from build123d import *

# Parameters (mm, degrees)
SKETCH_1_R          = 25
EXTRUDE_1_DEPTH     = 80
CUT_EXTRUDE_1_DEPTH = 2


with BuildPart() as part:
    # 草图1 → 凸台-拉伸1 (new body)
    with BuildSketch(Plane.XY):
        Circle(SKETCH_1_R)
    extrude(amount=EXTRUDE_1_DEPTH)

    # 草图2 → 切除-拉伸1 (cut)
    with BuildSketch(Plane(origin=(0, 0, 0), x_dir=(-1, 0, 0), z_dir=(0, 0, -1))):
        with BuildLine():
            Line((19.074750083, -11.012812095), (21.650635095, -12.5))
            ThreePointArc((21.650635095, -12.5), (-4.010605572, -24.676203982), (-24.494897428, -5))
            ThreePointArc((-24.494897428, -5), (-15.811388301, 9.364916731), (0, 15))
            ThreePointArc((0, 15), (16.128487869, 6.826744229), (19.074750083, -11.012812095))
        make_face()
    extrude(amount=-CUT_EXTRUDE_1_DEPTH, mode=Mode.SUBTRACT)


solid = part.part
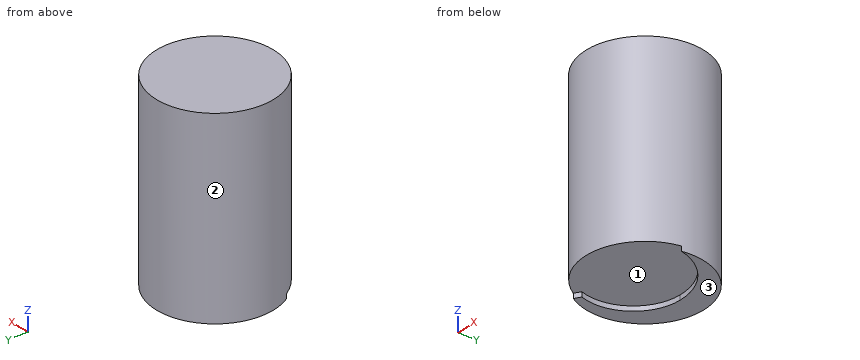
Model file for the job. Use its own axes, mm. Face numbers are marked on the shaded views. Give positions to 0.01 mm unless a question says otherwise; leave off trailing zeros. Loops run counter-clockwise (first coordinate to the right, second up) from the corner with the lowest first, then second, coordinate; pieces in that order, holes last.
1) Wall check: line 1 (Z direction, x = 8, y = 10.5); line 2 (Y direction, x = 0, z = 60); line 3 (X direction, y = -1, z = 29.5). Give the ranges that are in metal, low to high.
2) Saw through at B-B (x = 7). Write the cut outline in (y, z).
3) Saw through at C-C (z = 61). Write the cut outline in (x, y), plus the area to 3 significant figures.
4) Saw through at D-D (y = 12.5). Write the cut outline in (x, z), plus the area to 3 significant figures.
5) Flat gauge pins, fed straight in: pin 1 Ø1.5 at (x, y) = (-9, 1) entering from -Z; pin 2 Ø1 at (y, z) = (-6.5, 28.5) entering from +X; pin 3 Ø1.5 at (x, z) = (12, 16.5) entering from +Y. Where does each tip first touch, or does it go through?
6) Pull direction X, two halves, no side cores. Call the marked faces 1, 2 and 3: +X half, -X half, draft (parallel to the pull), parting line (faces both ways), or undercut.
7) Saw through at A-A (y = 0). Write the cut outline in (x, z).
Answer block:
1. line 1: z = 2 to 80
1. line 2: y = -25 to 25
1. line 3: x = -24.98 to 24.98
2. outline: (-24, 2) - (14, 2) - (14, 0) - (24, 0) - (24, 80) - (-24, 80) - close
3. outline: circle Ø50 at (0, 0)
3. area: 1,960 mm2
4. outline: (-21.65, 0) - (-9.68, 0) - (-9.68, 2) - (10.9, 2) - (10.9, 0) - (21.65, 0) - (21.65, 80) - (-21.65, 80) - close
4. area: 3,420 mm2
5. pin 1: stops at z = 2
5. pin 2: stops at x = 24.27
5. pin 3: stops at y = 22.33
6. face 1: undercut
6. face 2: parting line
6. face 3: draft
7. outline: (-25, 0) - (-19.36, 0) - (-19.36, 2) - (22.91, 2) - (22.91, 0) - (25, 0) - (25, 80) - (-25, 80) - close
